Build history of the part. All positions in model axes, mm. A direction names the side the tool comes from. Coordinates: 2 decimals unless noted, no trailing zeros. Order: outer loops, then holes, each group sorted by start corner. A loop starts at its lowest first (then second) coordinate and runs counter-clockwise, first axis right, second up. Notation, with made-up numbers: (11.5, -4.5) - (67.5, -4.5) arc R18 cw to (67.5, -0.5) - close; hole circle Ø11 at (51, 81). An arc over 180 degrees is marked (long way). Return JSON: item names as keys, results as strings.
from build123d import *

# Parameters (mm, degrees)
PAD_DEPTH            = 15
SKETCH001_W          = 7
SKETCH001_H          = 20
POCKET_DEPTH         = 97.489094
POCKET_DEPTH_BACK    = 97.489094
SKETCH002_R          = 1.5
POCKET001_DEPTH      = 109.489094
POCKET001_DEPTH_BACK = 109.489094


with BuildPart() as part:
    # Sketch (on DatumPlane) → Pad (new body, symmetric)
    with BuildSketch(Plane.XZ):
        with BuildLine():
            ThreePointArc((-15, 3), (-18, 0), (-15, -3))
            Line((-15, -3), (15, -3))
            ThreePointArc((15, -3), (18, 0), (15, 3))
            Line((-15, 3), (15, 3))
        make_face()
    extrude(amount=PAD_DEPTH, both=True)

    # Sketch001 (on DatumPlane) → Pocket (cut, two sides)
    with BuildSketch(Plane.XY) as pocket_sk:
        with Locations((-14.5, 0)):
            Rectangle(SKETCH001_W, SKETCH001_H)
    pocket = extrude(amount=-POCKET_DEPTH, mode=Mode.SUBTRACT) + extrude(pocket_sk.sketch, amount=POCKET_DEPTH_BACK, mode=Mode.SUBTRACT)

    # Mirrored: Pocket across YZ
    add(pocket.mirror(Plane.YZ), mode=Mode.SUBTRACT)

    # Sketch002 (on DatumPlane) → Pocket001 (cut, two sides)
    with BuildSketch(Plane.XZ) as pocket001_sk:
        with Locations((-15, 0)):
            Circle(SKETCH002_R)
    pocket001 = extrude(amount=-POCKET001_DEPTH, mode=Mode.SUBTRACT) + extrude(pocket001_sk.sketch, amount=POCKET001_DEPTH_BACK, mode=Mode.SUBTRACT)

    # Mirrored001: Pocket001 across YZ
    add(pocket001.mirror(Plane.YZ), mode=Mode.SUBTRACT)


solid = part.part
1. Cut at D-D on z = -2.6. Give the cut face in (x, y), plus the area to 3 significant figures.
Check values:
{"outline": "(-16.5, -15) - (16.5, -15) - (16.5, -10) - (11, -10) - (11, 10) - (16.5, 10) - (16.5, 15) - (-16.5, 15) - (-16.5, 10) - (-11, 10) - (-11, -10) - (-16.5, -10) - close", "area": "770 mm²"}
2. Probe L1, parallel to X at y = -11.55, z = 0; L2, parallel to X at y = -13, z = -0.4; L3, parallel to Y at x = 13.5, z = -0.9. List the from-to ranges inside material, lowest first.
Check values:
{"L1": "-18 to -16.5, -13.5 to 13.5, 16.5 to 18", "L2": "-17.97 to -16.45, -13.55 to 13.55, 16.45 to 17.97", "L3": "-15 to -10, 10 to 15"}
3. Cut at A-A on z = 0. Give the cut face in (x, y), plus the area to 3 significant figures.
Check values:
{"outline": "(-18, -15) - (-16.5, -15) - (-16.5, -10) - (-18, -10) - close; (-18, 10) - (-16.5, 10) - (-16.5, 15) - (-18, 15) - close; (-13.5, -15) - (13.5, -15) - (13.5, -10) - (11, -10) - (11, 10) - (13.5, 10) - (13.5, 15) - (-13.5, 15) - (-13.5, 10) - (-11, 10) - (-11, -10) - (-13.5, -10) - close; (16.5, -15) - (18, -15) - (18, -10) - (16.5, -10) - close; (16.5, 10) - (18, 10) - (18, 15) - (16.5, 15) - close", "area": "740 mm²"}
4. Tool access for faces 1 (the flat face through (11, 0, 0)), 2 (the flat face through (-13, -10, 0)), 3 (the flat face through (0, -15, 0)): list every direction of +Z, -Z, +X, -X, +Y, -Y with a clear straight run to the whole face (end or side of a thin tool).
Check values:
{"face 1": "+Z, -Z, +X", "face 2": "+Z, -Z, -X", "face 3": "+Z, -Z, +X, -X, -Y"}
5. Drop flat-ended pins along their axis: pin 1 (1.8 mm diameter, centred on x = 15, z = 0, fed in from +Y); pin 2 (1 mm diameter, centred on y = -11, z = -2.5, fed in from +X). Give the stop position or say it passes through.
Check values:
{"pin 1": "through", "pin 2": "x = 17.24"}
6. Cut at B-B on y = 11. Give the cut face in (x, z), plus the area to 3 significant figures.
Check values:
{"outline": "(-15, -3) - (15, -3) arc R3 ccw to (15, 3) - (-15, 3) arc R3 ccw to start; hole circle Ø3 at (-15, 0); hole circle Ø3 at (15, 0)", "area": "194 mm²"}
7. Cut at C-C on x = 15.5. Give the cut face in (y, z).
Check values:
{"outline": "(-15, -2.96) - (-10, -2.96) - (-10, -1.41) - (-15, -1.41) - close; (-15, 1.41) - (-10, 1.41) - (-10, 2.96) - (-15, 2.96) - close; (10, -2.96) - (15, -2.96) - (15, -1.41) - (10, -1.41) - close; (10, 1.41) - (15, 1.41) - (15, 2.96) - (10, 2.96) - close"}
8. Mould opens along X. For faces 4 (the flat face through (0, 15, 0)), 5 (the cylindrical face through (18, -13, 0)), 6 (the cylindrical face through (-18, -13, 0)), 7 (the cylindrical face through (-16.5, 12.46, 0.07)) say: pulls with the +X half, pulls with the -X half, needs draft (parallel to the pull), parting line crosses it, or undercut.
Check values:
{"face 4": "needs draft", "face 5": "pulls with the +X half", "face 6": "pulls with the -X half", "face 7": "undercut"}
